The listing builds one solid part. Answer for the finished solid, in the listing's coordinates (mm). Give positions to 0.01 mm unless a question says otherwise; leave off trailing zeros. Order: outer loops, then holes, each group sorted by start corner. A loop starts at its lowest first (then second) coordinate and runs counter-clockwise, first axis right, second up. Notation, with made-up numbers: (-17.5, -6) - (29.5, -6) arc R37 cw to (29.5, 30) - close; hole circle Ø1 at (40.25, -13.75). An arc over 180 degrees is marked (long way). Answer in a Markdown table with one row per item.
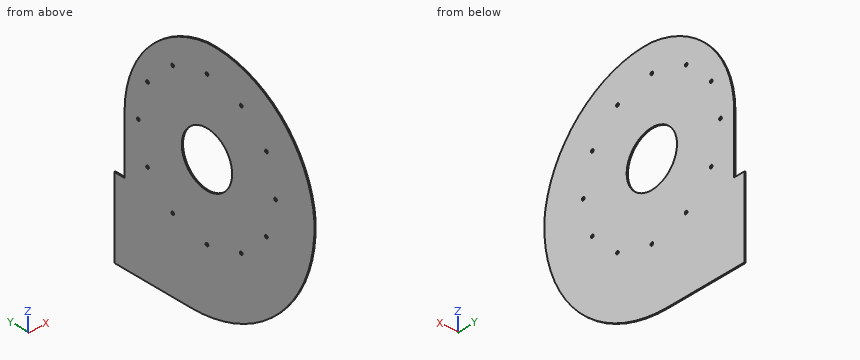
from build123d import *

# Parameters (mm, degrees)
SKETCH1_R           = 110
BOSS_EXTRUDE1_DEPTH = 5
SKETCH2_R           = 6
CUT_EXTRUDE1_DEPTH  = 10
CIRPATTERN1_COUNT   = 12


with BuildPart() as part:
    # Sketch1 → Boss-Extrude1 (new body)
    with BuildSketch(Plane(origin=(0, 0, 0), x_dir=(0, 0, -1), z_dir=(1, 0, 0))):
        with BuildLine():
            Line((-126.985698369, 168.770507744), (193.014301631, 168.770507744))
            Line((193.014301631, 168.770507744), (193.014301631, -166.625210225))
            ThreePointArc((193.014301631, -166.625210225), (29.499330124, -553.664543235), (-361.985698369, -706.229492256))
            ThreePointArc((-361.985698369, -706.229492256), (-663.674001264, -555.574607548), (-771.985698369, -236.229492256))
            ThreePointArc((-771.985698369, -236.229492256), (-634.689640971, 20.877775707), (-361.985698369, 123.770507744))
            Line((-361.985698369, 123.770507744), (-126.985698369, 123.770507744))
            Line((-126.985698369, 123.770507744), (-126.985698369, 168.770507744))
        make_face()
        with Locations((-361.985698369, -236.229492256)):
            Circle(SKETCH1_R, mode=Mode.SUBTRACT)
    extrude(amount=BOSS_EXTRUDE1_DEPTH)

    # Sketch2 → Cut-Extrude1 (cut)
    with BuildSketch(Plane.ZY):
        with Locations((661.985698369, -236.229492256)):
            Circle(SKETCH2_R)
    cut_extrude1 = extrude(amount=-CUT_EXTRUDE1_DEPTH, mode=Mode.SUBTRACT)

    # CirPattern1: Cut-Extrude1 ×12 about axis
    cirpattern1_axis = Axis((0, -236.229492256, 361.985698369), (1, 0, 0))
    for i in range(1, CIRPATTERN1_COUNT):
        add(cut_extrude1.rotate(cirpattern1_axis, i * 360 / CIRPATTERN1_COUNT), mode=Mode.SUBTRACT)


solid = part.part
Item 1: Find section B-B on z = 643. Write down the section's boundary in (x, y), then the cut area to 3 significant figures.
Answer block:
| item | result |
|---|---|
| outline | (0, -577.7) - (5, -577.7) - (5, 13.38) - (0, 13.38) - close |
| area | 2,960 mm² |
Item 2: Consider line 1 (Z direction, x = 2.4, y = -325.5); line 2 (Y direction, x = 2.5, z = 396); line 3 (Y direction, x = 0.4, z = 61). Determine where each line is inside the solid, lowest interval first.
Answer block:
| item | result |
|---|---|
| line 1 | -169.11 to 297.71, 426.26 to 768.62 |
| line 2 | -702.42 to -340.84, -131.62 to 122.34 |
| line 3 | -624.58 to -242.15, -230.31 to 168.77 |
Item 3: Each of these flat-tipped pins is pushed along its axis until it touches: P1, Ø3, axis at x = 2, y = 6, coming from the +Z side; P2, Ø7, axis at y = -536.23, z = 361.99, coming from the -X side; P3, Ø1, axis at x = 3.5, y = -381, coming from the +Z side; P4, Ø2.5, axis at x = 3.5, y = 138.5, coming from the +Z side. Where does it stop, or does it pass through?
Answer block:
| item | result |
|---|---|
| P1 | z = 652.28 |
| P2 | through |
| P3 | z = 757.36 |
| P4 | z = 126.99 |
Item 4: Find section A-A on x = 1.4. Count the separate pieces of the cut face and the enclosed holes in it, then the cut area to 3 significant figures.
Answer block:
| item | result |
|---|---|
| separate pieces | 1 |
| enclosed holes | 13 |
| area | 637,000 mm² |
Item 5: Find section C-C on y = -456. Write down the section's boundary in (x, z).
Answer block:
| item | result |
|---|---|
| outline | (0, -108.9) - (5, -108.9) - (5, 729.25) - (0, 729.25) - close |
